Build history of the part. All positions in model axes, mm. Round coordinates to 2 decimals unless told otherwise and drop trailing zeros. Write each loop counter-clockwise with the first axis right and the second up, starting at its lowest first coordinate (ties: lowest second). Pieces come first, ordered by that corner, then holes. Notation, with made-up numbers: (55, 20.5) -> (74, 20.5) arc R13 ccw to (74, 28.5) -> close; hole circle Ø4 at (-12.5, 6.25). An arc over 180 degrees is marked (long way). Answer in a Markdown table with one row per item.
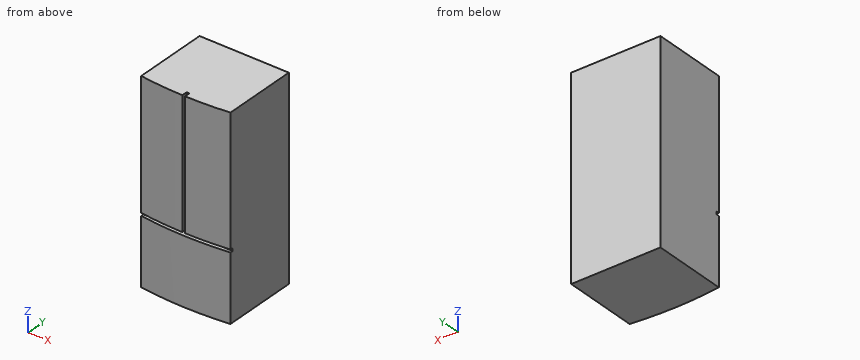
```python
from build123d import *

# Parameters (mm, degrees)
F1_DEPTH = 1803.4
F4_DEPTH = 50.8
F3_W     = 25.4
F3_H     = 2540
F5_DEPTH = 50.8


with BuildPart() as f1:
    # F0 (on Top) → F1 (new body)
    with BuildSketch(Plane.XY):
        with BuildLine():
            Line((407.9875, 714.375), (-407.9875, 714.375))
            Line((-407.9875, 714.375), (-407.9875, 25.4))
            ThreePointArc((-407.9875, 25.4), (0, 0), (407.9875, 25.4))
            Line((407.9875, 25.4), (407.9875, 714.375))
        make_face()
    extrude(amount=F1_DEPTH)

    # F2 (on Front) → F4 (cut)
    with BuildSketch(Plane.XZ):
        Polygon((-635, 635), (-635, 609.6), (0, 609.6), (635, 609.6), (635, 635), align=None)
    extrude(amount=-F4_DEPTH, mode=Mode.SUBTRACT)

    # F3 (on Front) → F5 (cut)
    with BuildSketch(Plane.XZ):
        with Locations((0, 1879.6)):
            Rectangle(F3_W, F3_H)
    extrude(amount=-F5_DEPTH, mode=Mode.SUBTRACT)


solid = f1.part
```
Q1. Saw through at B-B on x = -342. Write the cut outline in (y, z) (1 decimal).
A:
| item | result |
|---|---|
| outline | (17.8, 0) -> (714.4, 0) -> (714.4, 1803.4) -> (17.8, 1803.4) -> (17.8, 635) -> (50.8, 635) -> (50.8, 609.6) -> (17.8, 609.6) -> close |
Q2. Saw through at A-A on x = 271. Write the cut outline in (y, z) (3 decimals).
A:
| item | result |
|---|---|
| outline | (11.182, 0) -> (714.375, 0) -> (714.375, 1803.4) -> (11.182, 1803.4) -> (11.182, 635) -> (50.8, 635) -> (50.8, 609.6) -> (11.182, 609.6) -> close |
Q3. Wall check: line 1 (Z direction, x = -47, y = 41); line 2 (X direction, y = 49, z = 649.5); line 3 (Y direction, x = -12.5, z = 202.5) (3 decimals). Give the ranges that are in metal, low to high. Write a range as [from, to].
A:
| item | result |
|---|---|
| line 1 | [0, 609.6], [635, 1803.4] |
| line 2 | [-407.99, -12.7], [12.7, 407.99] |
| line 3 | [0.024, 714.375] |
